Could you check a few things on this model? Use its own coordinates, in mm. A direction names the side the tool comes from. Round coordinates to 2 decimals unless told otherwise and drop trailing zeros. Order: outer loops, then holes, each group sorted by start corner. A loop starts at its lowest first (then second) coordinate and runs counter-clockwise, first axis right, second up. Notation, with made-up numbers: (9.5, -12) -> (44.5, -12) arc R13 ccw to (44.5, 2) -> close; hole circle Ø8 at (64.25, 2). An arc over 180 degrees is marked (long way). Put each result on its own line as item: value. Start each with the question number.
from build123d import *

# Parameters (mm, degrees)
BOSS_EXTRUDE1_DEPTH     = 14
SKETCH2_R               = 4.75
BOSS_EXTRUDE2_DEPTH     = 1.5
SKETCH8_R               = 1.55
BOSS_EXTRUDE3_DEPTH     = 3
BOSS_EXTRUDE4_START     = -25.1
SKETCH8_2_R             = 1.55
BOSS_EXTRUDE4_DEPTH     = 3
BOSS_EXTRUDE6_DEPTH     = 12.6
M2_5_TAPPED_HOLE1_D     = 2.05
M2_5_TAPPED_HOLE1_DEPTH = 1.5
BOSS_EXTRUDE8_DEPTH     = 5
BOSS_EXTRUDE9_REACH     = 17.72
SKETCH22_W              = 4.537973116
SKETCH22_H              = 2
FILLET2_R               = 1
BOSS_EXTRUDE11_DEPTH    = 10.5
M3_TAPPED_HOLE2_D       = 2.5
M3_TAPPED_HOLE2_DEPTH   = 15.5
M3_TAPPED_HOLE2_TIP     = 0.751075774
BOSS_EXTRUDE12_DEPTH    = 9.6
SKETCH26_W              = 15
SKETCH26_H              = 3
BOSS_EXTRUDE13_DEPTH    = 12.7


with BuildPart() as part:
    # Sketch1 → Boss-Extrude1 (new body)
    with BuildSketch(Plane.XY):
        Polygon((9.075946232, 0), (4.537973116, 7.86), (-4.537973116, 7.86), (-9.075946232, 0), (-4.537973116, -7.86), (4.537973116, -7.86), align=None)
        Polygon((7.343895424, 0), (3.671947712, 6.36), (-3.671947712, 6.36), (-7.343895424, 0), (-3.671947712, -6.36), (3.671947712, -6.36), align=None, mode=Mode.SUBTRACT)
    extrude(amount=BOSS_EXTRUDE1_DEPTH)

    # Sketch2 → Boss-Extrude2 (add)
    with BuildSketch(Plane(origin=(0, 0, 0), x_dir=(-1, 0, 0), z_dir=(0, 0, -1))):
        Polygon((9.075946232, 0), (4.537973116, 7.86), (-4.537973116, 7.86), (-9.075946232, 0), (-4.537973116, -7.86), (4.537973116, -7.86), align=None)
        Circle(SKETCH2_R, mode=Mode.SUBTRACT)
    extrude(amount=BOSS_EXTRUDE2_DEPTH)

    # Sketch8 → Boss-Extrude3 (add)
    with BuildSketch(Plane.XY.offset(14)):
        Polygon((-7.5, -17.86), (7.5, -17.86), (7.5, -7.86), (9.075946232, -7.86), (9.075946232, 0), (4.537973116, -7.86), (-4.537973116, -7.86), (-9.075946232, 0), (-9.075946232, -7.86), (-7.5, -7.86), align=None)
        with Locations((-3.5, -13.91)):
            Circle(SKETCH8_R, mode=Mode.SUBTRACT)
        with Locations((3.5, -13.91)):
            Circle(SKETCH8_R, mode=Mode.SUBTRACT)
    extrude(amount=-BOSS_EXTRUDE3_DEPTH)



with BuildPart() as body_2:
    # Sketch8<2> → Boss-Extrude4 (new body)
    with BuildSketch(Plane.XY.offset(14).offset(BOSS_EXTRUDE4_START)):
        Polygon((-7.5, -7.86), (-7.5, -17.86), (7.5, -17.86), (7.5, -7.86), (7.5, -5.36), (5.981348789, -5.36), (4.537973116, -7.86), (-4.537973116, -7.86), (-5.981348789, -5.36), (-7.5, -5.36), align=None)
        with Locations((-3.5, -13.91)):
            Circle(SKETCH8_2_R, mode=Mode.SUBTRACT)
        with Locations((3.5, -13.91)):
            Circle(SKETCH8_2_R, mode=Mode.SUBTRACT)
    extrude(amount=-BOSS_EXTRUDE4_DEPTH)


with BuildPart() as part_1:
    add(part.part)

    add(body_2.part)  # Boss-Extrude6 merges body 2
    # Sketch9 → Boss-Extrude6 (add)
    with BuildSketch(Plane(origin=(0, 0, -1.5), x_dir=(-1, 0, 0), z_dir=(0, 0, -1))):
        Polygon((-5.981348789, -5.36), (5.981348789, -5.36), (4.537973116, -7.86), (-4.537973116, -7.86), align=None)
    extrude(amount=BOSS_EXTRUDE6_DEPTH)

    # M2.5 Tapped Hole1
    with Locations(Plane(origin=(0, 7.86, 0), x_dir=(1, 0, 0), z_dir=(0, 1, 0))):
        with Locations((0, -2.5), (0, -11.5)):
            Hole(M2_5_TAPPED_HOLE1_D / 2, depth=M2_5_TAPPED_HOLE1_DEPTH)

    # Sketch14 → Boss-Extrude8 (add)
    with BuildSketch(Plane.XY.offset(14)):
        Polygon((-4.537973116, 7.86), (-11.537973116, 7.86), (-11.537973116, -7.86), (-9.075946232, -7.86), (-9.075946232, 0), align=None)
        Polygon((9.075946232, -7.86), (9.075946232, 0), (4.537973116, 7.86), (11.537973116, 7.86), (11.537973116, -7.86), align=None)
    extrude(amount=-BOSS_EXTRUDE8_DEPTH)

    # Sketch22 → Boss-Extrude9 (add, up to next)
    with BuildSketch(Plane.XZ.offset(7.86), mode=Mode.PRIVATE) as boss_extrude9_sk1:
        with Locations((-6.806959674, 10)):
            Rectangle(SKETCH22_W, SKETCH22_H)
    boss_extrude9_tool1 = extrude(boss_extrude9_sk1.sketch, amount=-BOSS_EXTRUDE9_REACH, mode=Mode.PRIVATE) - part_1.part
    add(boss_extrude9_tool1.solids().sort_by_distance((-6.80696, -7.86, 10))[0])
    # Sketch22 → Boss-Extrude9 (add, up to next)
    with BuildSketch(Plane.XZ.offset(7.86), mode=Mode.PRIVATE) as boss_extrude9_sk2:
        with Locations((6.806959674, 10)):
            Rectangle(SKETCH22_W, SKETCH22_H)
    boss_extrude9_tool2 = extrude(boss_extrude9_sk2.sketch, amount=-BOSS_EXTRUDE9_REACH, mode=Mode.PRIVATE) - part_1.part
    add(boss_extrude9_tool2.solids().sort_by_distance((6.80696, -7.86, 10))[0])

    # Fillet2
    fillet2_edges = [part_1.edges().sort_by_distance(p)[0] for p in [
        (0, -5.36, -14.1),
    ]]
    fillet(fillet2_edges, radius=FILLET2_R)

    # Sketch24 → Boss-Extrude11 (add)
    with BuildSketch(Plane(origin=(0, 0, 9), x_dir=(-1, 0, 0), z_dir=(0, 0, -1))):
        Polygon((-11.537973116, -7.86), (-4.537973116, -7.86), (-9.075946232, 0), (-4.537973116, 7.86), (-11.537973116, 7.86), align=None)
        Polygon((4.537973116, 7.86), (9.075946232, 0), (4.537973116, -7.86), (11.537973116, -7.86), (11.537973116, 7.86), align=None)
    extrude(amount=BOSS_EXTRUDE11_DEPTH)

    # M3 Tapped Hole2
    with Locations(Plane.XY.offset(14)):
        with Locations((-8.105997779, 4.68), (-8.105997779, -4.68), (8.105997779, 4.68), (8.105997779, -4.68)):
            Hole(M3_TAPPED_HOLE2_D / 2, depth=M3_TAPPED_HOLE2_DEPTH)
            with Locations((0, 0, -(M3_TAPPED_HOLE2_DEPTH + M3_TAPPED_HOLE2_TIP / 2))):  # 118° drill point
                Cone(0, M3_TAPPED_HOLE2_D / 2, M3_TAPPED_HOLE2_TIP, mode=Mode.SUBTRACT)

    # Sketch25 → Boss-Extrude12 (add)
    with BuildSketch(Plane(origin=(0, 0, -1.5), x_dir=(-1, 0, 0), z_dir=(0, 0, -1))):
        Polygon((-5.981348789, -5.36), (-5.981348789, -7.86), (-4.537973116, -7.86), align=None)
    extrude(amount=BOSS_EXTRUDE12_DEPTH)

    # Sketch26 → Boss-Extrude13 (add)
    with BuildSketch(Plane.XZ.offset(17.86)):
        with Locations((0, 12.5)):
            Rectangle(SKETCH26_W, SKETCH26_H)
    extrude(amount=BOSS_EXTRUDE13_DEPTH)


solid = part_1.part
1. Which directions (+Z, -Z, +X, -X, +Y, -Y) give clear straight access to the entire face, cutting with the end or side of a thin tool? Please do faces 1 (the face through (5.981, -7, -6)), 2 (the face through (0, -17.86, -13)), 3 (the face through (0, -5.36, -7)), 4 (the face through (7.5, -19, 12)), 5 (the face through (5.482, -3.225, 6.902)).
2. Thinking about a two-plate mould opening in X: for faces 6 (the face through (0, -30.56, 13)), 7 (the face through (-7.5, -19, 12)), 8 (the face through (6.914, 5.055, 6.142)), which applies, +X half, -X half, draft (parallel to the pull), parting line (faces both ways), or undercut?
3. I need wall thicknesses on L1, parallel to Z at x = 0, y = 6.8 (3 decimals); L2, parallel to Y at x = 8.25, z = 6; L3, parallel to Y at x = -3, z = 7.75. Which ranges of each line are inside material? Lowest first, please.
4. For pin 1 Ø1.5 at (x, z) = (-7, 7) entering from -Y; pin 2 Ø2 at (x, y) = (-2, -25.5) entering from -Z; pin 3 Ø0.9 at (x, z) = (0.5, -12.5) entering from -Y, each with a flat end and sliding along its axis, tell me the tip position at first contact or that it passes through.
5. If we section it at A-A, the plane y = -13.91: Please give me the cut outline in (x, z), then the cut area to 3 significant figures.
6. If we section it at C-C, the plane z = 11.5: Please give me the cut outline in (x, y) (3 decimals), then the cut area to 3 significant figures.
7. If we section it at D-D, the plane y = 2: Please give me the cut outline in (x, z).
8. If we section it at B-B, the plane x = 0: Please give me the cut outline in (y, z) (3 decimals), then the cut area to 3 significant figures.
Results below:
1. face 1: +X, +Y, -Y
1. face 2: -Z, +X, -X, -Y
1. face 3: -Z, +X, -X, +Y
1. face 4: +Z, -Z, +X, -Y
1. face 5: +Z
2. face 6: draft
2. face 7: -X half
2. face 8: undercut
3. L1: -1.5 to 1.475, 3.525 to 10.475, 12.525 to 14
3. L2: -7.86 to -5.92, -3.44 to 3.44, 5.92 to 7.86
3. L3: -7.86 to -6.36, 6.36 to 7.86
4. pin 1: y = -7.86
4. pin 2: z = 11
4. pin 3: y = -17.86
5. outline: (-7.5, -14.1) -> (-5.05, -14.1) -> (-5.05, -11.1) -> (-7.5, -11.1) -> close; (-7.5, 11) -> (-5.05, 11) -> (-5.05, 14) -> (-7.5, 14) -> close; (-1.95, -14.1) -> (1.95, -14.1) -> (1.95, -11.1) -> (-1.95, -11.1) -> close; (-1.95, 11) -> (1.95, 11) -> (1.95, 14) -> (-1.95, 14) -> close; (5.05, -14.1) -> (7.5, -14.1) -> (7.5, -11.1) -> (5.05, -11.1) -> close; (5.05, 11) -> (7.5, 11) -> (7.5, 14) -> (5.05, 14) -> close
5. area: 52.8 mm2
6. outline: (-11.538, -7.86) -> (-7.5, -7.86) -> (-7.5, -30.56) -> (7.5, -30.56) -> (7.5, -7.86) -> (11.538, -7.86) -> (11.538, 7.86) -> (1.025, 7.86) -> (1.025, 6.36) -> (3.672, 6.36) -> (7.344, 0) -> (3.672, -6.36) -> (-3.672, -6.36) -> (-7.344, 0) -> (-3.672, 6.36) -> (-1.025, 6.36) -> (-1.025, 7.86) -> (-11.538, 7.86) -> close; hole circle Ø2.5 at (-8.106, -4.68); hole circle Ø2.5 at (-8.106, 4.68); hole circle Ø3.1 at (-3.5, -13.91); hole circle Ø3.1 at (3.5, -13.91); hole circle Ø2.5 at (8.106, -4.68); hole circle Ø2.5 at (8.106, 4.68)
6. area: 525 mm2
7. outline: (-11.54, -1.5) -> (-4.31, -1.5) -> (-4.31, 0) -> (-6.19, 0) -> (-6.19, 14) -> (-11.54, 14) -> close; (4.31, -1.5) -> (11.54, -1.5) -> (11.54, 14) -> (6.19, 14) -> (6.19, 0) -> (4.31, 0) -> close
8. outline: (-30.56, 11) -> (-7.86, 11) -> (-7.86, -11.1) -> (-17.86, -11.1) -> (-17.86, -14.1) -> (-6.36, -14.1) arc R1 ccw to (-5.36, -13.1) -> (-5.36, -1.5) -> (-4.75, -1.5) -> (-4.75, 0) -> (-6.36, 0) -> (-6.36, 14) -> (-30.56, 14) -> close; (4.75, -1.5) -> (7.86, -1.5) -> (7.86, 1.475) -> (6.36, 1.475) -> (6.36, 0) -> (4.75, 0) -> close; (6.36, 3.525) -> (7.86, 3.525) -> (7.86, 10.475) -> (6.36, 10.475) -> close; (6.36, 12.525) -> (7.86, 12.525) -> (7.86, 14) -> (6.36, 14) -> close
8. area: 175 mm2
